The model under review builds one solid part; all positions refer to its coordinate system, in mm. Coordinates: 2 decimals unless noted, no trailing zeros. Write each loop counter-clockwise with the first axis right and the second up, starting at its lowest first coordinate (ties: lowest second). Pieces come first, ordered by that corner, then holes. Notation, with made-up numbers: M 66,70 L 118,70 A26 ccw 118,106 Z; hole C -20,69 d6. An arc over 180 degrees is marked long. Answer as CSV lines item,"result". Start each with the question number.
Autodesk Inventor part; units mm, degrees
ref_plane "YZ Plane" through (0, 0, 0) normal (1, 0, 0) x (0, 1, 0)
ref_plane "XZ Plane" through (0, 0, 0) normal (0, 1, 0) x (-1, 0, 0)
ref_plane "XY Plane" through (0, 0, 0) normal (0, 0, 1) x (1, 0, 0)
sketch "Sketch1" plane through (0, 0, 0) normal (0, 0, 1) x (1, 0, 0)
  line L0 (0, 0) -> (6.35, 0)
  line L1 (6.35, 0) -> (6.35, 15.875)
  line L2 (6.35, 15.875) -> (0, 15.875)
  line L3 (0, 15.875) -> (0, 0)
  line L4 (3.175, 15.875) -> (3.175, 0) construction
  point P0 (3.175, 12.7)
  point P1 (3.175, 3.175)
  dimension "d0" = 6.35
  dimension "d1" = 15.875
  dimension "d2" = 3.175
  dimension "d3" = 3.175
extrude "Extrusion1" add sketch "Sketch1" along normal blind 6.35
hole "Hole1" at (3.175, 12.7, 0) at (3.175, 3.175, 0) direction (0, 0, 1) diameter 3.6576 end through all
sketch "Sketch2" plane through (0, 0, 0) normal (-1, 0, 0) x (0, 0, 1)
  line L0 (6.35, 15.875) -> (6.35, 0)
  line L1 (0, 15.875) -> (6.35, 15.875)
  point P0 (3.175, 7.9375)
  dimension "d13" = 3.175
  dimension "d14" = 7.9375
hole "Hole2" at (0, 7.9375, 3.175) direction (1, 0, 0) diameter 2.6416 end through all
properties part number "Cim Adjustment Block"
1) Mouldability with a two-part tool opening along Z and no side actions: class faces 1 (the flat face through (3, 0, 3)), 2 (the cylindrical face through (3.22, 6.63, 3)), 3 (the flat face through (3, 8, 0)), 4 (the flat face through (3, 8, 6.35)) as +Z half, -Z half, draft (parallel to the pull), parting line (faces both ways), or undercut.
2) To check wall thickness, follow line 1 (Y direction, x = 4, z = 1) (3 decimals); line 2 (Y direction, x = 3, z = 4.75) (3 decimals); line 3 (Y direction, x = 4, z = 3) (3 decimals). State the ranges of each line that lie inside material, in increasing order. Write a range as [from, to].
3) Take a section at B-B on z = 3.25. Give the boundary of the cut face in (x, y) (3 decimals).
4) Take a section at C-C on y = 12.7. Give the boundary of the cut face in (x, z).
5) Take a section at A-A on x = 3.75. Give the number of separate pieces and of enclosed holes in the cut face, and give its area (3 significant figures).
6) Clearance check with a flat-ended pin moving along its axis: pin 1 Ø1 at (y, z) = (6.5, 5.5) entering from -X. State where the tip first meets the part, or that it passes through.
Results:
1,face 1,"draft"
1,face 2,"undercut"
1,face 3,"-Z half"
1,face 4,"+Z half"
2,line 1,"y = [0, 1.543], [4.807, 11.068], [14.332, 15.875]"
2,line 2,"y = [0, 1.355], [4.995, 10.88], [14.52, 15.875]"
2,line 3,"y = [0, 1.543], [4.807, 6.628], [9.247, 11.068], [14.332, 15.875]"
3,outline,"M 0,0 L 6.35,0 L 6.35,6.619 L 0,6.619 Z; M 0,9.256 L 6.35,9.256 L 6.35,15.875 L 0,15.875 Z; hole C 3.175,3.175 d3.658; hole C 3.175,12.7 d3.658"
4,outline,"M 0,0 L 1.35,0 L 1.35,6.35 L 0,6.35 Z; M 5,0 L 6.35,0 L 6.35,6.35 L 5,6.35 Z"
5,separate pieces,"3"
5,enclosed holes,"1"
5,area,"51.2 mm²"
6,pin 1,"stops at x = 0"
